from build123d import *

# Parameters (mm, degrees)
SKETCH1_R           = 2
BOSS_EXTRUDE1_DEPTH = 3.5


with BuildPart() as part:
    # Sketch1 → Boss-Extrude1 (new body)
    with BuildSketch(Plane.XY.offset(13.5)):
        Polygon((-22.5, 18.556624327), (-20, 17.113248654), (-17.5, 18.556624327), (-17.5, 21.443375673), (-20, 22.886751346), (-22.5, 21.443375673), align=None)
        with Locations((-20, 20)):
            Circle(SKETCH1_R, mode=Mode.SUBTRACT)
    extrude(amount=-BOSS_EXTRUDE1_DEPTH)


solid = part.part
Source: CAD feature listing. Evaluate the final solid. Frame: model axes, mm. Round coordinates to 2 decimals unless told otherwise and drop trailing zeros. Order: outer loops, then holes, each group sorted by start corner. A loop starts at its lowest first (then second) coordinate and runs counter-clockwise, first axis right, second up. Notation, with made-up numbers: (38.25, -13) - (91.25, -13) arc R29 ccw to (91.25, 11) - close; hole circle Ø9 at (34.25, -19). An arc over 180 degrees is marked (long way). Use a Markdown table: item, result. Add a question column.
1. Section query A-A (y = 20). Return the cut outline in (x, z).
2. Mould query, pull axis X, two halves, no side actions, for faces 1 (the cylindrical face through (-20, 22, 12)), 2 (the flat face through (-21.268, 17.845, 11.774)), 3 (the flat face through (-18.732, 22.155, 11.774)). Classes: +X half, -X half, draft (parallel to the pull), parting line (faces both ways), or undercut.
3. Section query B-B (z = 11.85). Return the cut outline in (x, y).
4. Section query C-C (x = -21.55). Return the cut outline in (y, z).
5. First-contact query: pin 1 (1 mm diameter, centred on x = -19, y = 20, fed in from +Z). Flat tip, straight axial feed; report the tip coordinate or a pass-through.
6. Line query: probe 1 along Y at (x, z) = (-19.95, 11.25); probe 2 along X at (y, z) = (18.9, 12.9); probe 3 along Y at (x, z) = (-18.45, 10.6). Output: solid intervals per line, ascending.
7. Section query D-D (y = 17.7). Return the cut outline in (x, z), then the cut area to 3 significant figures.
Derived:
| question | item | result |
|---|---|---|
| 1 | outline | (-22.5, 10) - (-22, 10) - (-22, 13.5) - (-22.5, 13.5) - close; (-18, 10) - (-17.5, 10) - (-17.5, 13.5) - (-18, 13.5) - close |
| 2 | face 1 | undercut |
| 2 | face 2 | -X half |
| 2 | face 3 | +X half |
| 3 | outline | (-22.5, 18.56) - (-20, 17.11) - (-17.5, 18.56) - (-17.5, 21.44) - (-20, 22.89) - (-22.5, 21.44) - close; hole circle Ø4 at (-20, 20) |
| 4 | outline | (18.01, 10) - (18.74, 10) - (18.74, 13.5) - (18.01, 13.5) - close; (21.26, 10) - (21.99, 10) - (21.99, 13.5) - (21.26, 13.5) - close |
| 5 | pin 1 | through |
| 6 | probe 1 | 17.14 to 18, 22 to 22.86 |
| 6 | probe 2 | -22.5 to -21.67, -18.33 to -17.5 |
| 6 | probe 3 | 18.01 to 18.74, 21.26 to 21.99 |
| 7 | outline | (-21.02, 10) - (-18.98, 10) - (-18.98, 13.5) - (-21.02, 13.5) - close |
| 7 | area | 7.11 mm2 |
